Read the model definition and answer for the solid it produces. Units are mm, in the model's axes. A direction names the side the tool comes from. Give positions to 0.01 mm unless a question says otherwise; leave off trailing zeros. Write each loop counter-clockwise with the first axis right and the second up, starting at its lowest first coordinate (ties: lowest second). Pieces come first, ordered by that corner, then holes. Notation, with made-up numbers: (65, 35.5) - (107, 35.5) arc R29 ccw to (107, 68.5) - close; hole circle Ø8 at (77, 43.25). An arc over 180 degrees is marked (long way). Answer as a JSON object with one key per item and string values. Group by question number.
```python
from build123d import *

# Parameters (mm, degrees)
SKETCH1_W           = 12.7
SKETCH1_H           = 12.7
SKETCH1_W_2         = 9.398
SKETCH1_H_2         = 9.398
BOSS_EXTRUDE1_DEPTH = 101.6
SKETCH2_R           = 1.75
CUT_EXTRUDE1_DEPTH  = 22.2885
SKETCH3_R           = 1.75
CUT_EXTRUDE2_DEPTH  = 22.098
SKETCH4_R           = 1.75
CUT_EXTRUDE3_DEPTH  = 24.892


with BuildPart() as part:
    # Sketch1 → Boss-Extrude1 (new body)
    with BuildSketch(Plane(origin=(0, 0, 0), x_dir=(0, 1, 0), z_dir=(0, 0, 1))):
        Rectangle(SKETCH1_W, SKETCH1_H)
        Rectangle(SKETCH1_W_2, SKETCH1_H_2, mode=Mode.SUBTRACT)
    extrude(amount=BOSS_EXTRUDE1_DEPTH)

    # Sketch2 → Cut-Extrude1 (cut)
    with BuildSketch(Plane(origin=(0, 6.35, 0), x_dir=(-1, 0, 0), z_dir=(0, 1, 0))):
        with Locations(Location((-2.54, 80.9625, 0), (0, 0, 90))):
            Circle(SKETCH2_R)
        with Locations(Location((2.54, 71.4375, 0), (0, 0, 90))):
            Circle(SKETCH2_R)
        with Locations(Location((-2.54, 30.1625, 0), (0, 0, 90))):
            Circle(SKETCH2_R)
        with Locations(Location((2.54, 20.6375, 0), (0, 0, 90))):
            Circle(SKETCH2_R)
    extrude(amount=-CUT_EXTRUDE1_DEPTH, mode=Mode.SUBTRACT)

    # Sketch3 → Cut-Extrude2 (cut)
    with BuildSketch(Plane.YZ.offset(6.35)):
        with Locations(Location((-2.54, 14.2875, 0), (0, 0, 270))):
            Circle(SKETCH3_R)
        with Locations(Location((2.54, 4.7625, 0), (0, 0, 270))):
            Circle(SKETCH3_R)
        with Locations(Location((-2.54, 96.8375, 0), (0, 0, 270))):
            Circle(SKETCH3_R)
        with Locations(Location((2.54, 87.3125, 0), (0, 0, 270))):
            Circle(SKETCH3_R)
        with Locations(Location((-2.54, 58.7375, 0), (0, 0, 270))):
            Circle(SKETCH3_R)
        with Locations(Location((2.54, 49.2125, 0), (0, 0, 270))):
            Circle(SKETCH3_R)
    extrude(amount=-CUT_EXTRUDE2_DEPTH, mode=Mode.SUBTRACT)

    # Sketch4 → Cut-Extrude3 (cut)
    with BuildSketch(Plane(origin=(0, 6.35, 0), x_dir=(-1, 0, 0), z_dir=(0, 1, 0))):
        with Locations(Location((0, 9.525, 0), (0, 0, 90))):
            Circle(SKETCH4_R)
    extrude(amount=-CUT_EXTRUDE3_DEPTH, mode=Mode.SUBTRACT)


solid = part.part
```
1) Find the intervals of material crossed by line 1 (Z direction, x = 5.5, y = -2.75); line 2 (Z direction, x = 2.5, y = -4.75); line 3 (Y direction, x = 2.5, z = 34), in increasing order. Write a range as [from, to].
2) Which of the six approach directions +Z, -Z, +X, -X, +Y, -Y give full straight-line access (tool end or side, diameter ignored) to faces 1 (the flat face through (0, -4.699, 50)), 2 (the cylindrical face through (3.07, 5.54, 31.83))?
3) A flat-ended cylindrical pin translates along its axis: pin 1 Ø2 at (y, z) = (-2.54, 96.84) entering from +X. Find the tip coordinate at first contact, or state that the pin passes through.
4) Find section C-C, the plane z = 21. Write down the section's boundary in (x, y).
5) Find section A-A, the plane y = 2.54. Give the number of separate pieces and of enclosed holes in the cut face, and give its area (3 significant figures).
6) Find section B-B, the plane z = 91. Write down the section's boundary in (x, y).
7) For a pull along Y with two mould halves and no side action, classify faces 3 (the cylindrical face through (-5.513, -2.463, 60.486)), 4 (the cylindrical face through (-2, 5.5, 22.3)), 5 (the flat face through (0, 6.35, 50)) as released by +Y, released by -Y, zero draft, split by the parting line, or undercut.
Values follow:
{
 "1": {"line 1": "z = [0, 12.55], [16.02, 57], [60.47, 95.1], [98.57, 101.6]", "line 2": "z = [0, 28.41], [31.91, 79.21], [82.71, 101.6]", "line 3": "y = [-6.35, -4.7], [4.7, 6.35]"},
 "2": {"face 1": "+Z, -Z", "face 2": "+Y, -Y"},
 "3": {"pin 1": "passes through"},
 "4": {"outline": "(-6.35, -6.35) - (-4.25, -6.35) - (-4.25, -4.7) - (-4.7, -4.7) - (-4.7, 4.7) - (-4.25, 4.7) - (-4.25, 6.35) - (-6.35, 6.35) - close; (-0.83, -6.35) - (6.35, -6.35) - (6.35, 6.35) - (-0.83, 6.35) - (-0.83, 4.7) - (4.7, 4.7) - (4.7, -4.7) - (-0.83, -4.7) - close"},
 "5": {"separate pieces": "8", "enclosed holes": "0", "area": "301 mm2"},
 "6": {"outline": "(-6.35, -6.35) - (6.35, -6.35) - (6.35, 6.35) - (-6.35, 6.35) - close; hole (-4.7, -4.7) - (4.7, -4.7) - (4.7, 4.7) - (-4.7, 4.7) - close"},
 "7": {"face 3": "undercut", "face 4": "zero draft", "face 5": "released by +Y"}
}
